```python
from build123d import *

# Parameters (mm, degrees)
SKIZZE1_R                       = 50
SKIZZE1_R_2                     = 15
AUFSATZ_LINEAR_AUSTRAGEN1_DEPTH = 30
AUFSATZ_LINEAR_AUSTRAGEN2_DEPTH = 30
KREISMUSTER1_COUNT              = 18
SKIZZE3_R                       = 25
SCHNITT_LINEAR_AUSTRAGEN1_DEPTH = 5
SCHNITT_LINEAR_START            = -5
SKIZZE4_R                       = 25
SCHNITT_LINEAR_AUSTRAGEN2_DEPTH = 5


with BuildPart() as part:
    # Skizze1 → Aufsatz-Linear austragen1 (new body)
    with BuildSketch(Plane.XY):
        Circle(SKIZZE1_R)
        Circle(SKIZZE1_R_2, mode=Mode.SUBTRACT)
    extrude(amount=AUFSATZ_LINEAR_AUSTRAGEN1_DEPTH)

    # Skizze2 → Aufsatz-Linear austragen2 (add)
    with BuildSketch(Plane.XY.offset(30)):
        with BuildLine():
            Line((6, 46.636185446), (-6, 46.636185446))
            Line((-6, 46.636185446), (-4, 57.360700833))
            ThreePointArc((-4, 57.360700833), (0, 57.5), (4, 57.360700833))
            Line((4, 57.360700833), (6, 46.636185446))
        make_face()
    aufsatz_linear_austragen2 = extrude(amount=-AUFSATZ_LINEAR_AUSTRAGEN2_DEPTH)

    # Kreismuster1: Aufsatz-Linear austragen2 ×18 about axis
    kreismuster1_axis = Axis((0, 0, 0), (0, 0, 1))
    for i in range(1, KREISMUSTER1_COUNT):
        add(aufsatz_linear_austragen2.rotate(kreismuster1_axis, i * 360 / KREISMUSTER1_COUNT))

    # Skizze3 → Schnitt-Linear austragen1 (cut)
    with BuildSketch(Plane.XY.offset(30)):
        Circle(SKIZZE3_R)
    extrude(amount=-SCHNITT_LINEAR_AUSTRAGEN1_DEPTH, mode=Mode.SUBTRACT)

    # Skizze4 → Schnitt-Linear austragen2 (cut)
    with BuildSketch(Plane(origin=(0, 0, 0), x_dir=(-1, 0, 0), z_dir=(0, 0, -1)).offset(SCHNITT_LINEAR_START)):
        with Locations(Location((0, 0, 0), (0, 0, 180))):
            Circle(SKIZZE4_R)
    extrude(amount=SCHNITT_LINEAR_AUSTRAGEN2_DEPTH, mode=Mode.SUBTRACT)


solid = part.part
```
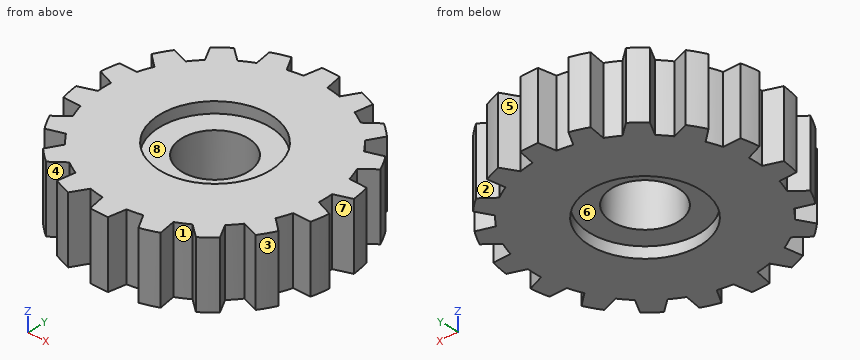
Geometry: final body of the model. Coordinates: model frame, mm. Face numbers are marked on the shaded views. A direction names the side the tool comes from. Coordinates: 2 decimals unless noted, no trailing zeros. Write each loop counter-clockwise with the first axis right and the second up, starting at its lowest first coordinate (ties: lowest second). Pieces come first, ordered by that corner, then holes. Notation, with made-up numbers: M 31.25,-21.75 L 49.25,-21.75 A4 cw 49.25,-15.75 Z; hole C 12.5,-19 d10. An arc over 180 degrees is marked long. Answer as CSV lines item,"result". Start each with the question number.
Q1. Cut plane C-C on x = -42. Return the cut outline in (y, z).
Q2. Cut plane B-B on x = 0. Return the cut outline in (y, z).
Q3. Cut plane A-A on y = 0. Return the cut outline in (x, z).
Q4. Mould query, pull axis Y, two halves, no side actions, for the marked faces 1, 2 and 3. Classes: released by +Y, released by -Y, zero draft, split by the parting line, or undercut.
Q5. Reachability of the marked faces 4, 5, 6, 7 and 8 from +Z, -Z, +X, -X, +Y, -Y: full face, straight path, thin tool, end or side. Return the list, or none.
Q6. Line query: line 1 (X direction, y = 42.5, z = 10.75); line 2 (Y direction, x = 0, z = 2.4); line 3 (X direction, y = -44.5, z = 28.75). Output: solid intervals per line, ascending. Write a range as from..to.
Q7. Pin query (flat end, axial travel): P1, Ø3, axis at x = -45.5, z = 3, coming from the -Y side; P2, Ø1, axis at x = 43, z = 13, coming from the -Y side; P3, Ø6, axis at x = -17.5, y = 4.5, coming from the +Z side; P4, Ø25, axis at x = 2, y = -1, coming from the -Z side. Return the tip coordinate at first contact, or that it passes through.
Findings below:
1,outline,"M -30.14,0 L 30.14,0 L 30.14,30 L -30.14,30 Z"
2,outline,"M -57.5,0 L -25,0 L -25,5 L -15,5 L -15,25 L -25,25 L -25,30 L -57.5,30 Z; M 15,5 L 25,5 L 25,0 L 57.5,0 L 57.5,30 L 25,30 L 25,25 L 15,25 Z"
3,outline,"M -50,0 L -25,0 L -25,5 L -15,5 L -15,25 L -25,25 L -25,30 L -50,30 Z; M 15,5 L 25,5 L 25,0 L 50,0 L 50,30 L 25,30 L 25,25 L 15,25 Z"
4,face 1,"undercut"
4,face 2,"released by +Y"
4,face 3,"released by -Y"
5,face 4,"+Z, -Z, -Y"
5,face 5,"+Z, -Z, +Y"
5,face 6,"-Z"
5,face 7,"+Z, -Z, +X"
5,face 8,"+Z"
6,line 1,"x = -38.73..-28.93, -26.34..26.34, 28.93..38.73"
6,line 2,"y = -57.5..-25, 25..57.5"
6,line 3,"x = -36.41..-31.36, -22.8..22.8, 31.36..36.41"
7,P1,"stops at y = -31.91"
7,P2,"stops at y = -30.67"
7,P3,"stops at z = 25"
7,P4,"passes through"
